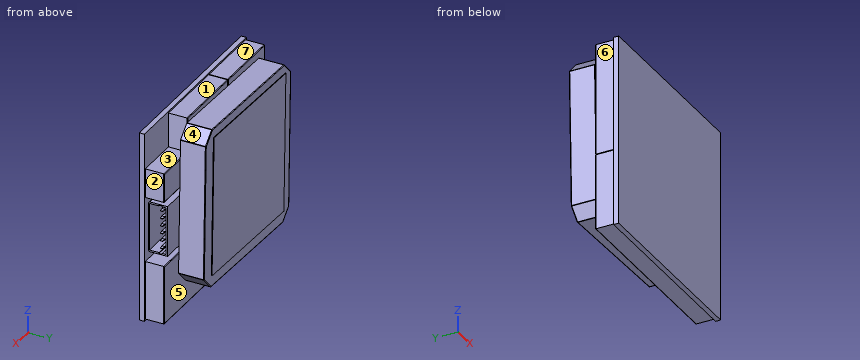
```python
from build123d import *
from OCP.BRepFilletAPI import BRepFilletAPI_MakeChamfer

# Parameters (mm, degrees)
SKETCH1_W           = 30.1
SKETCH1_H           = 30.1
BOSS_EXTRUDE1_DEPTH = 0.8
SKETCH2_W           = 10.771359077
SKETCH2_H           = 17.6
BOSS_EXTRUDE2_DEPTH = 3
FILLET1_R           = 0.1
SKETCH3_W           = 0.393223552
SKETCH3_H           = 8
BOSS_EXTRUDE3_DEPTH = 3
BOSS_EXTRUDE4_DEPTH = 5
SKETCH5_W           = 0.139227725
SKETCH5_H           = 0.457931022
BOSS_EXTRUDE5_DEPTH = 5
CHAMFER1_SIZE       = 0.05
CHAMFER1_SIZE2      = 0.571502615
BOSS_EXTRUDE6_DEPTH = 4
BOSS_EXTRUDE7_DEPTH = 0.1
FILLET2_R           = 0.1


with BuildPart() as part:
    # Sketch1 → Boss-Extrude1 (new body)
    with BuildSketch(Plane(origin=(0, 0, 0), x_dir=(1, 0, 0), z_dir=(0, 1, 0))):
        with Locations((15.05, 15.05)):
            Rectangle(SKETCH1_W, SKETCH1_H)
    extrude(amount=BOSS_EXTRUDE1_DEPTH)

    # Sketch2 → Boss-Extrude2 (add)
    with BuildSketch(Plane(origin=(0, 0.8, 0), x_dir=(1, 0, 0), z_dir=(0, 1, 0))):
        Polygon((29.85, 29.85), (0.25, 29.85), (0.25, 17.95), (11.121359077, 17.95), (11.121359077, 0.25), (23.021359077, 0.25), (23.021359077, 5.7), (29.85, 5.7), (29.85, 10.3), (23.021359077, 10.3), (23.021359077, 20.6), (29.85, 20.6), align=None)
        with Locations((5.635679539, 9.05)):
            Rectangle(SKETCH2_W, SKETCH2_H)
    extrude(amount=BOSS_EXTRUDE2_DEPTH)

    # Fillet1
    fillet1_edges = [part.edges().sort_by_distance(p)[0] for p in [
        (29.85, 3.8, -25.225),
        (15.05, 3.8, -29.85),
        (0.25, 3.8, -23.9),
        (5.685679539, 3.8, -17.95),
        (11.121359077, 3.8, -9.1),
        (17.071359077, 3.8, -0.25),
        (23.021359077, 3.8, -2.975),
        (26.435679539, 3.8, -5.7),
        (29.85, 3.8, -8),
        (26.435679539, 3.8, -10.3),
        (23.021359077, 3.8, -15.45),
        (26.435679539, 3.8, -20.6),
        (11.021359077, 3.8, -9.05),
        (5.635679539, 3.8, -17.85),
        (0.25, 3.8, -9.05),
        (5.635679539, 3.8, -0.25),
    ]]
    fillet(fillet1_edges, radius=FILLET1_R)

    # Sketch3 → Boss-Extrude3 (add)
    with BuildSketch(Plane(origin=(0, 0.8, 0), x_dir=(1, 0, 0), z_dir=(0, 1, 0))):
        with Locations((23.705954143, 15.45)):
            Rectangle(SKETCH3_W, SKETCH3_H)
    extrude(amount=BOSS_EXTRUDE3_DEPTH)

    # Sketch4 → Boss-Extrude4 (add)
    with BuildSketch(Plane(origin=(23.902565919, 0, 0), x_dir=(0, 0, -1), z_dir=(1, 0, 0))):
        Polygon((11.45, 3.8), (19.45, 3.8), (19.45, 0.954176152), (19.310192822, 0.8), (11.645064396, 0.8), (11.45, 0.976884701), align=None)
        Polygon((11.7, 3.55), (19.2, 3.55), (19.2, 2.943906616), (19.339550272, 2.943906616), (19.339550272, 2.443906616), (19.2, 2.443906616), (19.2, 0.954176152), (11.7, 0.954176152), (11.7, 2.443906616), (11.560449728, 2.443906616), (11.560449728, 2.943906616), (11.7, 2.943906616), align=None, mode=Mode.SUBTRACT)
    extrude(amount=BOSS_EXTRUDE4_DEPTH)

    # Sketch5 → Boss-Extrude5 (add)
    with BuildSketch(Plane(origin=(23.902565919, 0, 0), x_dir=(0, 0, -1), z_dir=(1, 0, 0))):
        with Locations((13.629724037, 2.842775415)):
            Rectangle(SKETCH5_W, SKETCH5_H)
        with Locations((12.429724037, 2.842775415)):
            Rectangle(SKETCH5_W, SKETCH5_H)
        with Locations((14.829724037, 2.842775415)):
            Rectangle(SKETCH5_W, SKETCH5_H)
        with Locations((16.029724036, 2.842775415)):
            Rectangle(SKETCH5_W, SKETCH5_H)
        with Locations((17.229724037, 2.842775415)):
            Rectangle(SKETCH5_W, SKETCH5_H)
        with Locations((18.429724037, 2.842775415)):
            Rectangle(SKETCH5_W, SKETCH5_H)
    extrude(amount=BOSS_EXTRUDE5_DEPTH)

    # Chamfer1: one chamfer whose edges measure the first distance from different faces: ONE call of the kernel's chamfer builder (chamfer() names one face for all edges)
    chamfer1_edges_1 = [part.edges().sort_by_distance(p)[0] for p in [
        (28.902565919, 2.842775415, -12.360110174),
        (28.902565919, 2.613809904, -12.429724036),
        (28.902565919, 2.842775415, -12.499337899),
        (28.902565919, 3.071740926, -12.429724036),
    ]]
    chamfer1_side_1 = [part.faces().sort_by_distance(p)[0] for p in [
        (28.902565919, 2.842775415, -12.429724036),
    ]]
    chamfer1_edges_2 = [part.edges().sort_by_distance(p)[0] for p in [
        (28.902565919, 2.842775415, -13.560110174),
        (28.902565919, 2.613809904, -13.629724036),
        (28.902565919, 2.842775415, -13.699337899),
        (28.902565919, 3.071740926, -13.629724036),
    ]]
    chamfer1_side_2 = [part.faces().sort_by_distance(p)[0] for p in [
        (28.902565919, 2.842775415, -13.629724036),
    ]]
    chamfer1_edges_3 = [part.edges().sort_by_distance(p)[0] for p in [
        (28.902565919, 2.842775415, -14.760110174),
        (28.902565919, 2.613809904, -14.829724036),
        (28.902565919, 2.842775415, -14.899337899),
        (28.902565919, 3.071740926, -14.829724036),
    ]]
    chamfer1_side_3 = [part.faces().sort_by_distance(p)[0] for p in [
        (28.902565919, 2.842775415, -14.829724036),
    ]]
    chamfer1_edges_4 = [part.edges().sort_by_distance(p)[0] for p in [
        (28.902565919, 2.842775415, -15.960110174),
        (28.902565919, 2.613809904, -16.029724036),
        (28.902565919, 2.842775415, -16.099337899),
        (28.902565919, 3.071740926, -16.029724036),
    ]]
    chamfer1_side_4 = [part.faces().sort_by_distance(p)[0] for p in [
        (28.902565919, 2.842775415, -16.029724036),
    ]]
    chamfer1_edges_5 = [part.edges().sort_by_distance(p)[0] for p in [
        (28.902565919, 2.842775415, -17.160110174),
        (28.902565919, 2.613809904, -17.229724036),
        (28.902565919, 2.842775415, -17.299337899),
        (28.902565919, 3.071740926, -17.229724036),
    ]]
    chamfer1_side_5 = [part.faces().sort_by_distance(p)[0] for p in [
        (28.902565919, 2.842775415, -17.229724036),
    ]]
    chamfer1_edges_6 = [part.edges().sort_by_distance(p)[0] for p in [
        (28.902565919, 2.842775415, -18.360110174),
        (28.902565919, 2.613809904, -18.429724036),
        (28.902565919, 2.842775415, -18.499337899),
        (28.902565919, 3.071740926, -18.429724036),
    ]]
    chamfer1_side_6 = [part.faces().sort_by_distance(p)[0] for p in [
        (28.902565919, 2.842775415, -18.429724036),
    ]]
    chamfer1 = BRepFilletAPI_MakeChamfer(part.part.solid().wrapped)
    for e in chamfer1_edges_1:
        chamfer1.Add(CHAMFER1_SIZE, CHAMFER1_SIZE2, e.wrapped, chamfer1_side_1[0].wrapped)  # the first distance lies on this face
    for e in chamfer1_edges_2:
        chamfer1.Add(CHAMFER1_SIZE, CHAMFER1_SIZE2, e.wrapped, chamfer1_side_2[0].wrapped)  # the first distance lies on this face
    for e in chamfer1_edges_3:
        chamfer1.Add(CHAMFER1_SIZE, CHAMFER1_SIZE2, e.wrapped, chamfer1_side_3[0].wrapped)  # the first distance lies on this face
    for e in chamfer1_edges_4:
        chamfer1.Add(CHAMFER1_SIZE, CHAMFER1_SIZE2, e.wrapped, chamfer1_side_4[0].wrapped)  # the first distance lies on this face
    for e in chamfer1_edges_5:
        chamfer1.Add(CHAMFER1_SIZE, CHAMFER1_SIZE2, e.wrapped, chamfer1_side_5[0].wrapped)  # the first distance lies on this face
    for e in chamfer1_edges_6:
        chamfer1.Add(CHAMFER1_SIZE, CHAMFER1_SIZE2, e.wrapped, chamfer1_side_6[0].wrapped)  # the first distance lies on this face
    add(Compound.cast(chamfer1.Shape()), mode=Mode.REPLACE)

    # Sketch6 → Boss-Extrude6 (add)
    with BuildSketch(Plane(origin=(0, 3.8, 0), x_dir=(1, 0, 0), z_dir=(0, 1, 0))):
        Polygon((2.384156778, 26.595544695), (23.597073632, 26.020012034), (25.660080778, 23.841939144), (25.08668319, 2.707716574), (23.200865717, 0.921525239), (1.93262783, 1.498558828), (0, 3.5389804), (0.579168662, 24.885912571), align=None)
    extrude(amount=BOSS_EXTRUDE6_DEPTH)

    # Sketch7 → Boss-Extrude7 (add)
    with BuildSketch(Plane(origin=(0, 7.8, 0), x_dir=(1, 0, 0), z_dir=(0, 1, 0))):
        Polygon((2.259866972, 24.824959048), (23.462598641, 24.249702724), (22.868758373, 2.362006201), (1.666026705, 2.937262525), align=None)
    extrude(amount=BOSS_EXTRUDE7_DEPTH)

    # Fillet2
    fillet2_edges = [part.edges().sort_by_distance(p)[0] for p in [
        (2.384156778, 5.8, -26.595544695),
        (0.579168662, 5.8, -24.885912571),
        (0, 5.8, -3.5389804),
        (1.93262783, 5.8, -1.498558828),
        (23.200865717, 5.8, -0.921525239),
        (25.08668319, 5.8, -2.707716574),
        (25.660080778, 5.8, -23.841939144),
        (23.597073632, 5.8, -26.020012034),
        (1.48166272, 7.8, -25.740728633),
        (0.289584331, 7.8, -14.212446486),
        (0.966313915, 7.8, -2.518769614),
        (12.566746773, 7.8, -1.210042034),
        (24.143774453, 7.8, -1.814620907),
        (25.373381984, 7.8, -13.274827859),
        (24.628577205, 7.8, -24.930975589),
        (12.990615205, 7.8, -26.307778365),
    ]]
    fillet(fillet2_edges, radius=FILLET2_R)


solid = part.part
```
Here's how the part is built. I have some questions about the finished solid (model axes, mm). Face numbers are marked on the shaded views. A direction names the side the tool comes from. Give positions to 0.01 mm unless a question says otherwise; leave off trailing zeros. Loops run counter-clockwise (first coordinate to the right, second up) from the corner with the lowest first, then second, coordinate; pieces in that order, holes last. Notation, with made-up numbers: M -39,67.5 L -4,67.5 A8 cw -4,75.5 Z; hole C 30,57.5 d9. An arc over 180 degrees is marked long. Put each result on its own line as item: value. Start each with the question number.
(1) I want a section at A-A on y = 2. Please give me the cut outline in (x, z), then the cut area to 3 significant figures.
(2) If we mould it in two halves opening along Y, with no side actions, what happens to the marked faces 5, 6 and 7? For each: +Y half, -Y half, draft (parallel to the pull), parting line (faces both ways), or undercut.
(3) I need wall thicknesses on line 1 along Z through (x, y) = (27, 3.5); line 2 along Z through (x, y) = (20, 3); line 3 along Y through (x, z) = (23.5, -3). Which ranges of each line are inside material? Lowest first, please. Write a range as [from, to].
(4) I want a section at C-C on z = -15.5. State how many separate pieces and enclosed holes the cut face has, then the cut area to 3 significant figures.
(5) Will these pins go through, and if not, where does the flat tip stop? pin 1 Ø2 at (y, z) = (7, -5) entering from -X; pin 2 Ø3 at (y, z) = (2.5, -26.5) entering from -X; pin 3 Ø0.9 at (x, y) = (26.5, 3) entering from +Z.
(6) I want a section at B-B on y = 6.5. Please give me the cut outline in (x, z).
(7) For the marked faces 1, 2, 3 and 4, which set-ups out of +Z, -Z, +X, -X, +Y, -Y let a thin tool reach every point of the face, with its end or its side?
Answer block:
1. outline: M 0.25,-29.85 L 29.85,-29.85 L 29.85,-20.6 L 23.02,-20.6 L 23.02,-10.3 L 29.85,-10.3 L 29.85,-5.7 L 23.02,-5.7 L 23.02,-0.25 L 11.12,-0.25 L 11.12,-17.95 L 0.25,-17.95 Z; M 0.25,-17.85 L 11.02,-17.85 L 11.02,-0.25 L 0.25,-0.25 Z; M 23.51,-19.45 L 28.9,-19.45 L 28.9,-19.2 L 23.9,-19.2 L 23.9,-11.7 L 28.9,-11.7 L 28.9,-11.45 L 23.51,-11.45 Z
1. area: 771 mm^2
2. face 5: +Y half
2. face 6: undercut
2. face 7: draft
3. line 1: [-29.85, -20.6], [-19.45, -19.2], [-11.7, -11.45], [-10.3, -5.7]
3. line 2: [-29.85, -0.25]
3. line 3: [0, 0.8], [3.8, 7.8]
4. separate pieces: 1
4. enclosed holes: 2
4. area: 198 mm^2
5. pin 1: x = 0.01
5. pin 2: x = 0.25
5. pin 3: z = -5.7
6. outline: M 0,-3.58 L 0.58,-24.84 A0.1 ccw 0.61,-24.91 L 2.35,-26.57 A0.1 ccw 2.43,-26.59 L 23.56,-26.02 A0.1 ccw 23.63,-25.99 L 25.63,-23.87 A0.1 ccw 25.66,-23.8 L 25.09,-2.75 A0.1 ccw 25.06,-2.68 L 23.23,-0.95 A0.1 ccw 23.16,-0.92 L 1.97,-1.5 A0.1 ccw 1.9,-1.53 L 0.03,-3.51 A0.1 ccw Z
7. face 1: +Z, +X, -X, +Y
7. face 2: +Z, -Z, +X, +Y
7. face 3: +Z, +X
7. face 4: +Z, +X, +Y
